from build123d import *

# Parameters (mm, degrees)
F0_W     = 42
F0_H     = 13
F0_R     = 1.65
F1_DEPTH = 18
F2_R     = 5
F3_DEPTH = 13
F4_SIZE  = 2
F5_SIZE  = 1


with BuildPart() as f1:
    # F0 (on Top) → F1 (new body)
    with BuildSketch(Plane.XY):
        Rectangle(F0_W, F0_H)
        with Locations((-15.5, 2.5)):
            Circle(F0_R, mode=Mode.SUBTRACT)
        with Locations((15.5, 2.5)):
            Circle(F0_R, mode=Mode.SUBTRACT)
    extrude(amount=F1_DEPTH)

    # F2 (on face) → F3 (cut, through all)
    with BuildSketch(Plane.XZ.offset(6.5)):
        with Locations((6, 10)):
            Circle(F2_R)
    extrude(amount=-F3_DEPTH, mode=Mode.SUBTRACT)

    # F4
    f4_edges = [f1.edges().sort_by_distance(p)[0] for p in [
        (-21, 0, 18),
        (0, -6.5, 18),
        (21, 0, 18),
    ]]
    chamfer(f4_edges, length=F4_SIZE)

    # F5
    f5_edges = [f1.edges().sort_by_distance(p)[0] for p in [
        (0, 6.5, 18),
    ]]
    chamfer(f5_edges, length=F5_SIZE)


solid = f1.part
The model under review builds one solid part; all positions refer to its coordinate system, in mm. Coordinates: 2 decimals unless noted, no trailing zeros. Order: outer loops, then holes, each group sorted by start corner. A loop starts at its lowest first (then second) coordinate and runs counter-clockwise, first axis right, second up. Notation, with made-up numbers: (84, 81) -> (119, 81) arc R20 ccw to (119, 120) -> close; hole circle Ø4 at (63, -38.75). An arc over 180 degrees is marked (long way). Answer in a Markdown table with one row per item.
(1) Consider section C-C (y = 3.5). Write out the cut boundary in (x, z), plus the area to 3 significant figures.
Answers:
| item | result |
|---|---|
| outline | (-21, 0) -> (-16.81, 0) -> (-16.81, 18) -> (-19, 18) -> (-21, 16) -> close; (-14.19, 0) -> (14.19, 0) -> (14.19, 18) -> (-14.19, 18) -> close; (16.81, 0) -> (21, 0) -> (21, 16) -> (19, 18) -> (16.81, 18) -> close; hole circle Ø10 at (6, 10) |
| area | 579 mm² |
(2) Insertion check: pin 1 (2 mm diameter, centred on x = 15.5, y = 2.5, fed in from +Z). The pin has a flat end and moves straight along its axis. Give the tip position at first contact, or say it passes through.
Answers:
| item | result |
|---|---|
| pin 1 | through |
(3) Consider section A-A (z = 6). Write out the cut boundary in (x, y), plus the area to 3 significant figures.
Answers:
| item | result |
|---|---|
| outline | (-21, -6.5) -> (3, -6.5) -> (3, 6.5) -> (-21, 6.5) -> close; (9, -6.5) -> (21, -6.5) -> (21, 6.5) -> (9, 6.5) -> close; hole circle Ø3.3 at (-15.5, 2.5); hole circle Ø3.3 at (15.5, 2.5) |
| area | 451 mm² |
(4) Consider section B-B (x = -15.5). Write out the cut boundary in (y, z).
Answers:
| item | result |
|---|---|
| outline | (-6.5, 0) -> (0.85, 0) -> (0.85, 18) -> (-4.5, 18) -> (-6.5, 16) -> close; (4.15, 0) -> (6.5, 0) -> (6.5, 17) -> (5.5, 18) -> (4.15, 18) -> close |
(5) Consider section D-D (z = 10). Write out the cut boundary in (x, y).
Answers:
| item | result |
|---|---|
| outline | (-21, -6.5) -> (1, -6.5) -> (1, 6.5) -> (-21, 6.5) -> close; (11, -6.5) -> (21, -6.5) -> (21, 6.5) -> (11, 6.5) -> close; hole circle Ø3.3 at (-15.5, 2.5); hole circle Ø3.3 at (15.5, 2.5) |
(6) The part is to be moulded in two halves that separate along X. For faces 1 (the flat face through (21, 0, 8)), 2 (the cylindrical face through (-13.926, 2.996, 8.874)), 3 (the flat face through (-0.3, 6, 17.5)), say which applies: +X half, -X half, draft (parallel to the pull), parting line (faces both ways), or undercut.
Answers:
| item | result |
|---|---|
| face 1 | +X half |
| face 2 | undercut |
| face 3 | draft |
(7) Wall thickness on line 1 along Z through (x, y) = (6, -3); line 2 along X through (y, z) = (1.75, 9.75); line 3 along Y through (x, z) = (15.5, 13.5): over which ranges is each line inside the solid? List them lowest first.
Answers:
| item | result |
|---|---|
| line 1 | 0 to 5, 15 to 18 |
| line 2 | -21 to -16.97, -14.03 to 1.01, 10.99 to 14.03, 16.97 to 21 |
| line 3 | -6.5 to 0.85, 4.15 to 6.5 |
